Build history of the part. All positions in model axes, mm. A direction names the side the tool comes from. Round coordinates to 2 decimals unless told otherwise and drop trailing zeros. Order: outer loops, then holes, each group sorted by start corner. A loop starts at its lowest first (then second) coordinate and runs counter-clockwise, first axis right, second up. Notation, with made-up numbers: (83, -6) - (131, -6) arc R20 cw to (131, 32) - close; hole circle Ø4 at (1.5, -38). An arc over 180 degrees is marked (long way). Write each question's results on one line, items separated by ' | '. Start each with the question number.
```python
from build123d import *

# Parameters (mm, degrees)
F0_R     = 17.5
F1_DEPTH = 2
F2_R     = 14.5
F3_DEPTH = 5.5
F4_W     = 5.75
F4_H     = 5.75
F5_DEPTH = 2
F8_R     = 1.6
F9_DEPTH = 6.5
F10_SIZE = 1.99999


# Not quite as in the source:
# - a fillet or chamfer is up to 0.001 mm smaller than in the source, because OpenCascade refuses the exact size


with BuildPart() as f1:
    # F0 (on Top) → F1 (new body)
    with BuildSketch(Plane.XY):
        Circle(F0_R)
    extrude(amount=F1_DEPTH)

    # F2 (on face) → F3 (join)
    with BuildSketch(Plane.XY.offset(2)):
        Circle(F2_R)
    extrude(amount=F3_DEPTH)


with BuildPart() as f5:
    # F4 (on face) → F5 (new body)
    with BuildSketch(Plane.XY.offset(7.5)):
        with BuildLine():
            Line((-2.875, 2.875), (2.875, 2.875))
            Line((2.875, 2.875), (2.875, 14.2121207073))
            ThreePointArc((2.875, 14.2121207073), (0, 14.5), (-2.875, 14.2121207073))
            Line((-2.875, 14.2121207073), (-2.875, 2.875))
        make_face()
        Rectangle(F4_W, F4_H)
    extrude(amount=F5_DEPTH)


with BuildPart() as f5_1:
    # F6: moved
    add(f5.part.moved(Location((0, 0, -4))))


with BuildPart() as f1_1:
    add(f1.part)

    # F7: cut F5
    add(f5_1.part, mode=Mode.SUBTRACT)

    # F8 (on face) → F9 (cut)
    with BuildSketch(Plane.XY.offset(7.5)):
        Circle(F8_R)
    extrude(amount=-F9_DEPTH, mode=Mode.SUBTRACT)

    # F10 (size 2 in the source; OpenCascade refuses exactly that, so slightly less here)
    f10_edges = [f1_1.edges().sort_by_distance(p)[0] for p in [
        (-17.5, 0, 0),
    ]]
    chamfer(f10_edges, length=F10_SIZE)


solid = f1_1.part
```
1. Flat gauge pins, fed straight in: pin 1 Ø1.5 at (x, z) = (4.5, 3.5) entering from +Y; pin 2 Ø1 at (x, z) = (0.5, 4.5) entering from +Y (3 decimals); pin 3 Ø4 at (x, z) = (-2, 4.5) entering from +Y. Where does each tip first touch, or does it go through?
2. Wall check: line 1 (Y direction, x = 0, z = 2.55); line 2 (X direction, y = 11, z = 3.75) (3 decimals); line 3 (Z direction, x = 0, y = -1). Give the ranges that are in metal, low to high. Write a range as from..to.
3. Cut at C-C (z = 3). List the corners of the cut face in (x, y), plus the area to 3 significant figures.
4. 3-axis set-ups, long thin cutter, end or side, ignore diameter. For faces 1 (the face through (0, 6, 3.5)), 2 (the face through (3, 0, 7.5)), 3 (the face through (-7, 13, 2)): which of +Z, -Z, +X, -X, +Y, -Y reach the whole face in a straight line?
5. Cut at D-D (z = 5). List the corners of the cut face in (x, y) (3 decimals).
6. Mould opens along Y. For faces 4 (the face through (6.691, -12.864, 4.712)), 5 (the face through (-1.27, -0.97, 6.51)), 6 (the face through (0, -2.875, 4)), 7 (the face through (0, 0, 0)) say: pulls with the +Y half, pulls with the -Y half, needs draft (parallel to the pull), parting line crosses it, or undercut.
A:
1) pin 1: stops at y = 14.01 | pin 2: stops at y = -2.875 | pin 3: stops at y = 14.5
2) line 1: y = -14.5..-1.6, 1.6..14.5 | line 2: x = -9.447..-2.875, 2.875..9.447 | line 3: z = 0..1
3) outline: circle Ø29 at (0, 0); hole circle Ø3.2 at (0, 0) | area: 652 mm^2
4) face 1: +Y | face 2: +Z, +X, -X, +Y, -Y | face 3: +Z
5) outline: (-2.875, -2.875) - (-2.875, 14.212) arc R14.5 ccw (long way) to (2.875, 14.212) - (2.875, -2.875) - close
6) face 4: parting line crosses it | face 5: undercut | face 6: pulls with the +Y half | face 7: needs draft
